Design review of the part built by this model. Coordinates are the model's own, in mm. Face numbers are marked on the shaded views. A direction names the side the tool comes from. Coordinates: 2 decimals unless noted, no trailing zeros. Loops run counter-clockwise (first coordinate to the right, second up) from the corner with the lowest first, then second, coordinate; pieces in that order, holes last. Notation, with made-up numbers: (62, 23) -> (83, 23) arc R28 cw to (83, 42) -> close; hole circle Ø1 at (71, 2.5). An arc over 180 degrees is marked (long way). Use a Markdown table: item, result. Add a question column.
Q1. Take a section at B-B on y = 139.7. Write out the cut boundary in (x, z).
Q2. Take a section at A-A on z = -10. Write out the cut boundary in (x, y), plus the area to 3 significant figures.
Q3. Take a section at C-C on x = 4. Write out the cut boundary in (y, z), plus the area to 3 significant figures.
Q4. Draft analysis for pull direction X (two halves, no side actions). For the marked faces 3, 4 and 5, state which applies: pulls with the +X half, pulls with the -X half, needs draft (parallel to the pull), parting line crosses it, or undercut.
Q5. For probe 1 along Z at (x, y) = (3, 106.5); probe 2 along Z at (x, y) = (17.5, 228.6), list the stretches that pass through material, from the lowest coordinate up.
Q6. Take a section at D-D on z = 16.5. Write out the cut boundary in (x, y).
Q7. Clearance check with a flat-ended pin moving along its axis: pin 1 Ø1.5 at (y, z) = (192.5, -14) entering from +X. State where the tip first meets the part, or that it passes through.
Q8. For the marked faces 1 and 2, list the 3-axis set-ups (+Z, -Z, +X, -X, +Y, -Y) from which the entire face can be reached by the end or side of a thin tool; tool diameter is ignored.
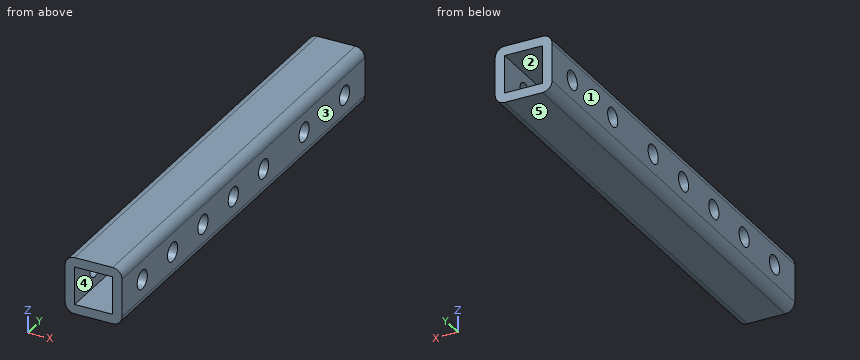
from build123d import *

# Parameters (mm, degrees)
F0_W     = 25.4
F0_H     = 25.4
F2_DEPTH = 304.8
F4_D     = 12.7
F1_D     = 12.7


with BuildPart() as f2:
    # F0 (on Front) → F2 (new body)
    with BuildSketch(Plane.XZ):
        with BuildLine():
            Line((-12.7, -19.05), (12.7, -19.05))
            ThreePointArc((12.7, -19.05), (17.190128, -17.190128), (19.05, -12.7))
            Line((19.05, -12.7), (19.05, 12.7))
            ThreePointArc((19.05, 12.7), (17.190128, 17.190128), (12.7, 19.05))
            Line((12.7, 19.05), (-12.7, 19.05))
            ThreePointArc((-12.7, 19.05), (-17.190128, 17.190128), (-19.05, 12.7))
            Line((-19.05, 12.7), (-19.05, -12.7))
            ThreePointArc((-19.05, -12.7), (-17.190128, -17.190128), (-12.7, -19.05))
        make_face()
        Rectangle(F0_W, F0_H, mode=Mode.SUBTRACT)
    extrude(amount=-F2_DEPTH)

    # F4 (through all)
    with Locations(Plane(origin=(0, 0, 0), x_dir=(0, 1, 0), z_dir=(-1, 0, 0))):
        with Locations((25.4, 0), (101.6, 0), (63.5, 0), (228.6, 0), (279.4, 0), (139.7, 0), (177.8, 0)):
            Hole(F4_D / 2)

    # F1 (through all)
    with Locations(Plane.YZ):
        with Locations((25.4, 0), (63.5, 0), (101.6, 0), (228.6, 0), (279.4, 0), (139.7, 0), (177.8, 0)):
            Hole(F1_D / 2)


solid = f2.part
Answer list:
| question | item | result |
|---|---|---|
| 1 | outline | (-19.05, -12.7) arc R6.35 ccw to (-12.7, -19.05) -> (12.7, -19.05) arc R6.35 ccw to (19.05, -12.7) -> (19.05, -6.35) -> (12.7, -6.35) -> (12.7, -12.7) -> (-12.7, -12.7) -> (-12.7, -6.35) -> (-19.05, -6.35) -> close; (-19.05, 6.35) -> (-12.7, 6.35) -> (-12.7, 12.7) -> (12.7, 12.7) -> (12.7, 6.35) -> (19.05, 6.35) -> (19.05, 12.7) arc R6.35 ccw to (12.7, 19.05) -> (-12.7, 19.05) arc R6.35 ccw to (-19.05, 12.7) -> close |
| 2 | outline | (-19.05, 0) -> (-12.7, 0) -> (-12.7, 304.8) -> (-19.05, 304.8) -> close; (12.7, 0) -> (19.05, 0) -> (19.05, 304.8) -> (12.7, 304.8) -> close |
| 2 | area | 3,870 mm² |
| 3 | outline | (0, -19.05) -> (304.8, -19.05) -> (304.8, -12.7) -> (0, -12.7) -> close; (0, 12.7) -> (304.8, 12.7) -> (304.8, 19.05) -> (0, 19.05) -> close |
| 3 | area | 3,870 mm² |
| 4 | face 3 | pulls with the +X half |
| 4 | face 4 | undercut |
| 4 | face 5 | needs draft |
| 5 | probe 1 | -19.05 to -12.7, 12.7 to 19.05 |
| 5 | probe 2 | -16.86 to -6.35, 6.35 to 16.86 |
| 6 | outline | (-17.79, 0) -> (17.79, 0) -> (17.79, 304.8) -> (-17.79, 304.8) -> close |
| 7 | pin 1 | x = 19.03 |
| 8 | face 1 | +Z, -Z, -X, +Y, -Y |
| 8 | face 2 | +Y, -Y |
